Job drawing, mm, ordinate dimensions from the low corner. One solid piece. A direction names the side the tool comes from. Round coordinates to 2 decimals unless told otherwise and drop trailing zeros. Write each loop counter-clockwise with the first axis right and the second up, starting at its lowest first coordinate (ties: lowest second). Pieces come first, ordered by that corner, then holes. Notation, with made-up numbers: M 18.25,-24 L 55.25,-24 A16 cw 55.25,-4 Z; hole C 70.5,65.5 d11. An arc over 180 degrees is marked long. Answer as a JSON object with one key per item and string values. Group by question number.
1. Two-plate mould, pull along X, no slides. Class the marked faces 4, 5 and 6: +X half, -X half, draft (parallel to the pull), parting line (faces both ways), or undercut.
2. Drop flat-ended pins along their axis: pin 1 (7.5 mm diameter, centred on y = 29.5, z = 9, fed in from +X); pin 2 (1 mm diameter, centred on x = 57, z = 5, fed in from -Y) (1 decimal); pin 3 (8 mm diameter, centred on x = 13.5, z = 4, fed in from +Y) (1 decimal). Give the stop position or say it passes through.
3. Drill centre lines: line 1 (X direction, y = 43.5, z = 15.25); line 2 (Y direction, x = 57.5, z = 15.5) (1 decimal); line 3 (X direction, y = 81, z = 15). Where is each one in solid material? Low to high. Write a range as from..to.
4. Band-saw the part on B-B, the plane x = 11.5. Write the cut outline in (y, z) (1 decimal), plus the area to 3 significant figures.
5. Band-saw the part on C-C, the plane y = 28. Write the cut outline in (x, z).
6. Which spindle directions (+Z, -Z, +X, -X, +Y, -Y) get a long thin tool onto all of the face, cutting with end or side? Do the marked faces 1, 2 and 3. Say none if no direction does.
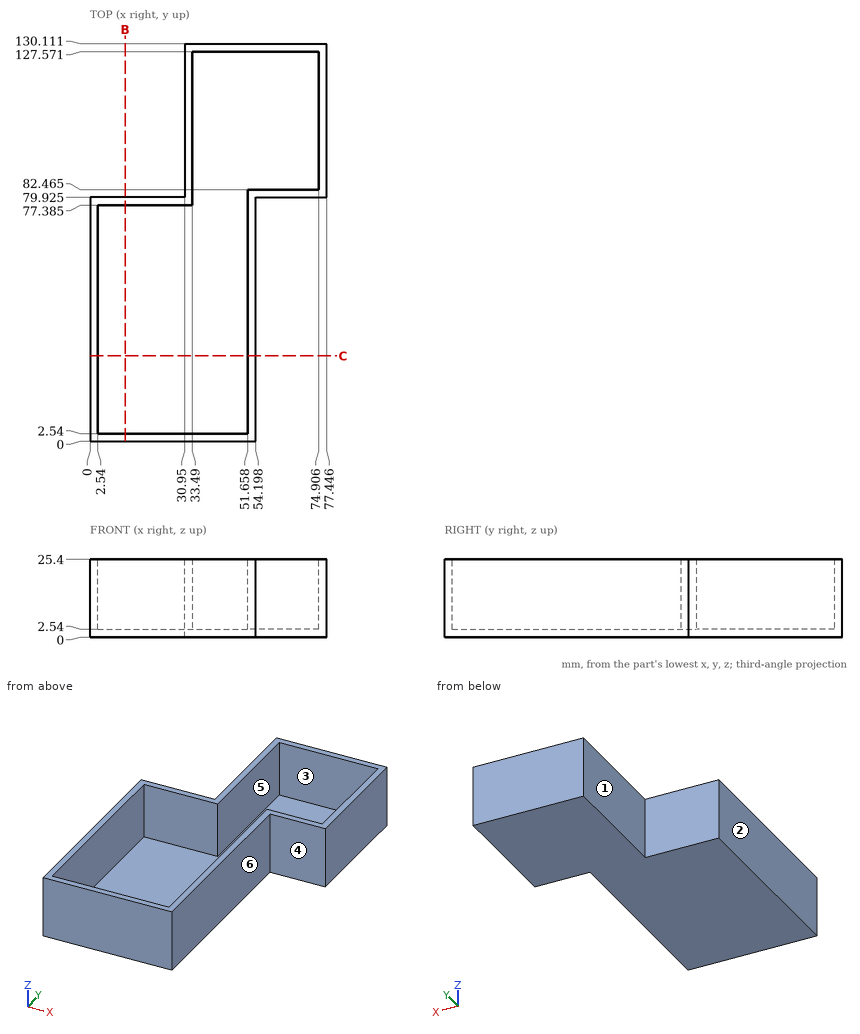
Worked answers:
{
 "1": {"face 4": "draft", "face 5": "undercut", "face 6": "+X half"},
 "2": {"pin 1": "stops at x = 54.2", "pin 2": "stops at y = 79.9", "pin 3": "stops at y = 79.9"},
 "3": {"line 1": "x = 0..2.54, 51.66..54.2", "line 2": "y = 79.9..82.5, 127.6..130.1", "line 3": "x = 30.95..33.49, 51.66..77.45"},
 "4": {"outline": "M 0,0 L 79.9,0 L 79.9,25.4 L 77.4,25.4 L 77.4,2.5 L 2.5,2.5 L 2.5,25.4 L 0,25.4 Z", "area": "319 mm^2"},
 "5": {"outline": "M 0,0 L 54.2,0 L 54.2,25.4 L 51.66,25.4 L 51.66,2.54 L 2.54,2.54 L 2.54,25.4 L 0,25.4 Z"},
 "6": {"face 1": "+Z, -Z, -X, +Y", "face 2": "+Z, -Z, -X, +Y, -Y", "face 3": "+Z"}
}
